```python
from build123d import *

# Parameters (mm, degrees)
SKETCH_1_W                 = 24
SKETCH_1_H                 = 24
SKETCH_1_W_2               = 20
SKETCH_1_H_2               = 20
EXTRUDE_1_DEPTH            = 4
SKETCH_6_R                 = 2
EXTRUDE_2_DEPTH            = 4
CHAMFER_1_SIZE             = 1
CHAMFER_1_OF_MIRROR_1_SIZE = 1


with BuildPart() as part:
    # Эскиз1 → Бобышка-Вытянуть1 (new body)
    with BuildSketch(Plane.XY):
        Rectangle(SKETCH_1_W, SKETCH_1_H)
        Rectangle(SKETCH_1_W_2, SKETCH_1_H_2, mode=Mode.SUBTRACT)
    extrude(amount=EXTRUDE_1_DEPTH)

    # Эскиз6 → Бобышка-Вытянуть2 (add)
    with BuildSketch(Plane(origin=(0, 12, 0), x_dir=(1, 0, 0), z_dir=(0, 1, 0))):
        with BuildLine():
            Line((-12, 2), (-18, 2))
            ThreePointArc((-18, 2), (-19.414213562, 1.414213562), (-20, 0))
            Line((-20, 0), (-20, -4))
            ThreePointArc((-20, -4), (-19.414213562, -5.414213562), (-18, -6))
            Line((-18, -6), (-12, -6))
            Line((-12, -6), (-12, 2))
        make_face()
        with Locations(Location((-16, -2, 0), (0, 0, 270))):
            Circle(SKETCH_6_R, mode=Mode.SUBTRACT)
    extrude_2 = extrude(amount=-EXTRUDE_2_DEPTH)

    # Фаска1
    chamfer_1_edges = [part.edges().sort_by_distance(p)[0] for p in [
        (-12, 10, -2),
        (-12, 10, 6),
    ]]
    chamfer(chamfer_1_edges, length=CHAMFER_1_SIZE)

    # Зеркальное отражение1: Бобышка-Вытянуть2 across plane
    add(extrude_2.mirror(Plane(origin=(0, 0, 0), x_dir=(0, 0, 1), z_dir=(1, 0, 0))))

    # Фаска1 of Зеркальное отражение1
    chamfer_1_of_mirror_1_edges = [part.edges().sort_by_distance(p)[0] for p in [
        (12, 10, -2),
        (12, 10, 6),
    ]]
    chamfer(chamfer_1_of_mirror_1_edges, length=CHAMFER_1_OF_MIRROR_1_SIZE)


solid = part.part
```
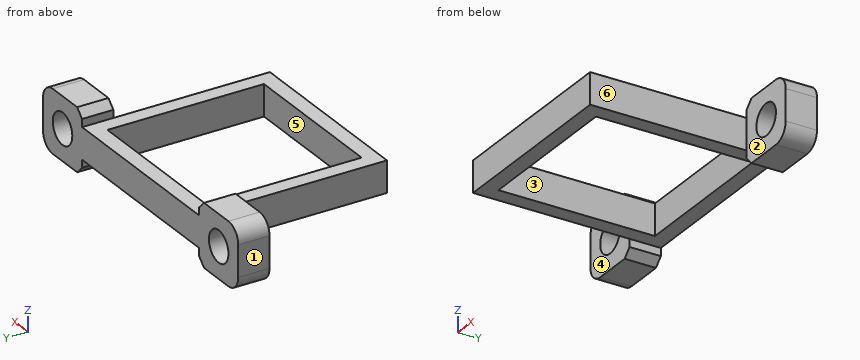
Check sheet for the modelled part. Datum: model origin and axes. Units: mm. Face numbers are marked on the shaded views. A direction names the side the tool comes from. Round coordinates to 2 decimals unless told otherwise and drop trailing zeros. Order: outer loops, then holes, each group sorted by start corner. A loop starts at its lowest first (then second) coordinate and runs counter-clockwise, first axis right, second up.
1) Tool access check on the marked faces 4, 5 and 6. Record the directions out of +Z, -Z, +X, -X, +Y, -Y that give a thin tool (end or side, any length) a straight path to the whole face; none if there is none.
2) Section check B-B (z = 2). Record the boundary of the cut face in (x, y).
3) Section check A-A (y = 1). Record the boundary of the cut face in (x, z).
4) Mould release check, pull along X, two halves, no side actions. Record for the marked faces 1, 2 and 3: +X half, -X half, draft (parallel to the pull), parting line (faces both ways), or undercut.
5) Section check C-C (x = -16). Record the boundary of the cut face in (y, z).
6) Scan lines: line 1 (X direction, y = 10.2, z = 2); line 2 (X direction, y = 9.7, z = 2); line 3 (Y direction, x = 2.5, z = 1). Record each from-to range of solid material in increasing order.
7) Section check D-D (x = 11). Record the boundary of the cut face in (y, z), and give its area (3 significant figures).
8) Go/stop test with flat-tipped pins: pin 1 Ø3 at (y, z) = (-1, 2.5) entering from -X; pin 2 Ø2 at (y, z) = (-4, 1.5) entering from +X; pin 3 Ø0.8 at (y, z) = (9, -0.5) entering from +X; pin 4 Ø2.5 at (x, z) = (-16, 2) entering from -Y. Record where each tip stops, or that it passes through.
Result:
1. face 4: +Z, -Z, -X, -Y
1. face 5: +Z, -Z
1. face 6: +Z, -Z, +X, -Y
2. outline: (-20, 8) - (-18, 8) - (-18, 12) - (-20, 12) - close; (-14, 8) - (-12, 8) - (-12, -12) - (12, -12) - (12, 8) - (14, 8) - (14, 12) - (-14, 12) - close; (18, 8) - (20, 8) - (20, 12) - (18, 12) - close; hole (-10, -10) - (10, -10) - (10, 10) - (-10, 10) - close
3. outline: (-12, 0) - (-10, 0) - (-10, 4) - (-12, 4) - close; (10, 0) - (12, 0) - (12, 4) - (10, 4) - close
4. face 1: -X half
4. face 2: draft
4. face 3: undercut
5. outline: (8, -2) - (12, -2) - (12, 0) - (8, 0) - close; (8, 4) - (12, 4) - (12, 6) - (8, 6) - close
6. line 1: x = -20 to -18, -14 to 14, 18 to 20
6. line 2: x = -20 to -18, -14 to -10, 10 to 14, 18 to 20
6. line 3: y = -12 to -10, 10 to 12
7. outline: (-12, 0) - (12, 0) - (12, 4) - (-12, 4) - close
7. area: 96.0 mm2
8. pin 1: stops at x = -12
8. pin 2: stops at x = 12
8. pin 3: stops at x = 20
8. pin 4: passes through
